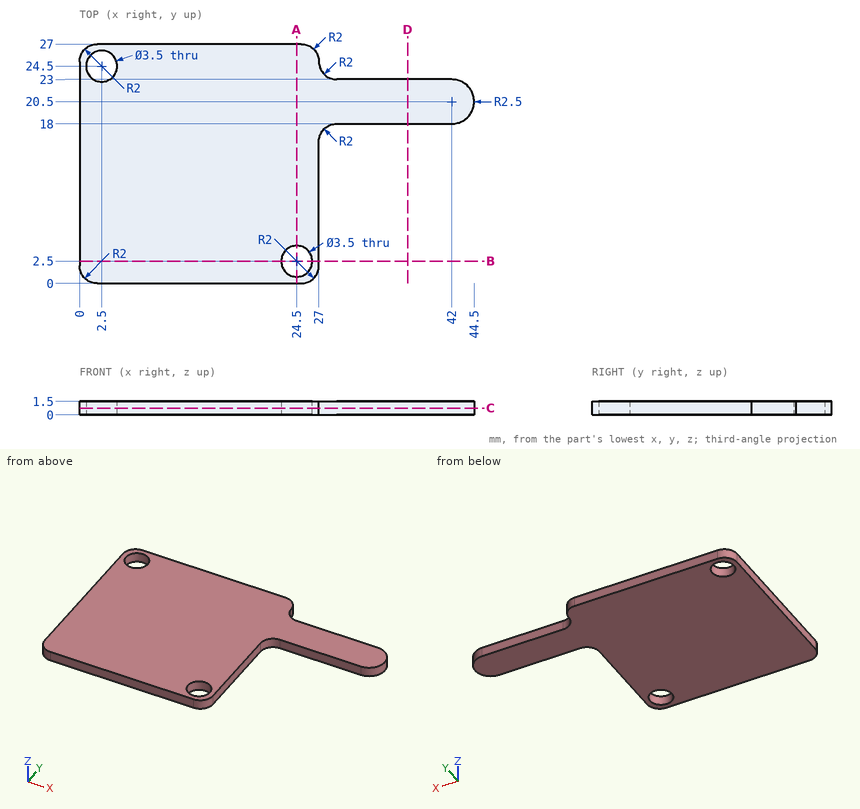
The figure shows three views and two pictorial views of one solid part (mm, origin at its lowest corner). Answer the questions. Coordinates: 2 decimals unless noted, no trailing zeros. Write each loop counter-clockwise with the first axis right and the second up, starting at its lowest first coordinate (ties: lowest second). Pieces come first, ordered by that corner, then holes. Notation, with made-up numbers: (84.25, -7) -> (111.25, -7) arc R22 ccw to (111.25, 9) -> close; hole circle Ø5 at (-38.75, -14). An arc over 180 degrees is marked (long way). Return JSON: item names as keys, results as strings.
(1) Consider line 1 along Y through (x, z) = (24.5, 0.35); line 2 along X through (y, z) = (7.25, 0.75); line 3 along Y through (x, z) = (2.5, 0.85). Determine where each line is inside the solid, lowest interval first. Write a range as from..to.
Answers below:
{"line 1": "0..0.75, 4.25..27", "line 2": "0..27", "line 3": "0..22.75, 26.25..27"}
(2) This flat-tipped pin is pushed along its axis until it touches: P1, Ø5, axis at x = 9, y = 6.5, coming from the -Z side. Where does it stop, or does it pass through?
Answers below:
{"P1": "z = 0"}
(3) The part is cut by section C-C on z = 0.75. State how many separate pieces and enclosed holes the cut face has, then the cut area to 3 significant figures.
Answers below:
{"separate pieces": "1", "enclosed holes": "2", "area": "793 mm^2"}
(4) The part is cut by section D-D on x = 37. Give the vertices of the cut face in (y, z).
Answers below:
{"outline": "(18, 0) -> (23, 0) -> (23, 1.5) -> (18, 1.5) -> close"}
(5) The part is cut by section B-B on y = 2.5. Give the vertices of the cut face in (x, z).
Answers below:
{"outline": "(0, 0) -> (22.75, 0) -> (22.75, 1.5) -> (0, 1.5) -> close; (26.25, 0) -> (27, 0) -> (27, 1.5) -> (26.25, 1.5) -> close"}
(6) The part is cut by section A-A on x = 24.5. Give the vertices of the cut face in (y, z).
Answers below:
{"outline": "(0, 0) -> (0.75, 0) -> (0.75, 1.5) -> (0, 1.5) -> close; (4.25, 0) -> (27, 0) -> (27, 1.5) -> (4.25, 1.5) -> close"}
